Here's how the part is built. I have some questions about the finished solid (model axes, mm). A direction names the side the tool comes from. Round coordinates to 2 decimals unless told otherwise and drop trailing zeros. Loops run counter-clockwise (first coordinate to the right, second up) from the corner with the lowest first, then second, coordinate; pieces in that order, holes last. Notation, with made-up numbers: M 25,9.25 L 71,9.25 A30 cw 71,41.25 Z; hole C -4,57 d9. An arc over 180 degrees is marked long. Answer as a JSON object with one key per item and string values.
from build123d import *

# Parameters (mm, degrees)
EXTRUSION1_DEPTH = 87.5
ESQUISSE3_R      = 1.5
EXTRUSION3_DEPTH = 10
ESQUISSE4_W      = 18.5
ESQUISSE4_H      = 20
EXTRUSION4_DEPTH = 1.5


with BuildPart() as part:
    # Esquisse1 → Extrusion1 (new body)
    with BuildSketch(Plane.XY):
        Polygon((0, 0), (20, 0), (20, 1.5), (1.5, 1.5), (1.5, 20), (0, 20), align=None)
    extrude(amount=EXTRUSION1_DEPTH)

    # Esquisse3 → Extrusion3 (cut)
    with BuildSketch(Plane.ZY):
        with Locations(Location((77.5, 10, 0), (0, 0, 270))):
            Circle(ESQUISSE3_R)
        with Locations(Location((10, 10, 0), (0, 0, 270))):
            Circle(ESQUISSE3_R)
    extrude(amount=-EXTRUSION3_DEPTH, mode=Mode.SUBTRACT)

    # Esquisse4 → Extrusion4 (cut)
    with BuildSketch(Plane.XZ):
        with Locations((10.75, 10)):
            Rectangle(ESQUISSE4_W, ESQUISSE4_H)
        with Locations((10.75, 77.5)):
            Rectangle(ESQUISSE4_W, ESQUISSE4_H)
    extrude(amount=-EXTRUSION4_DEPTH, mode=Mode.SUBTRACT)


solid = part.part
Item 1: For faces 1 (the face through (11, 1, 67.5)), 2 (the face through (20, 1, 43)), 3 (the face through (11, 1, 20)), which set-ups out of +Z, -Z, +X, -X, +Y, -Y let a thin tool reach every point of the face, with its end or its side?
Solution:
{"face 1": "+Z, +X, +Y, -Y", "face 2": "+Z, -Z, +X, +Y, -Y", "face 3": "-Z, +X, +Y, -Y"}
Item 2: I want a section at A-A on y = 10. List the corners of the cut face in (x, z) for me.
Solution:
{"outline": "M 0,0 L 1.5,0 L 1.5,8.5 L 0,8.5 Z; M 0,11.5 L 1.5,11.5 L 1.5,76 L 0,76 Z; M 0,79 L 1.5,79 L 1.5,87.5 L 0,87.5 Z"}
Item 3: I want a section at B-B on z = 77.5. List the corners of the cut face in (x, y) for me, plus the area to 3 significant figures.
Solution:
{"outline": "M 0,0 L 1.5,0 L 1.5,8.5 L 0,8.5 Z; M 0,11.5 L 1.5,11.5 L 1.5,20 L 0,20 Z", "area": "25.5 mm2"}
Item 4: For P1, Ø1.6, axis at x = 7.5, y = 1, coming from the -Z side; P2, Ø4, axis at y = 4, z = 77.5, coming from the +X side; P3, Ø9, axis at x = 8.5, z = 54.5, coming from the +Y side, each with a flat end and sliding along its axis, tell me the tip position at first contact or that it passes through.
Solution:
{"P1": "stops at z = 20", "P2": "stops at x = 1.5", "P3": "stops at y = 1.5"}
Item 5: I want a section at C-C on x = 7.5. List the corners of the cut face in (y, z) for me, plus the area to 4 significant figures.
Solution:
{"outline": "M 0,20 L 1.5,20 L 1.5,67.5 L 0,67.5 Z", "area": "71.25 mm2"}
Item 6: We'd pull the mould along Z, two halves only. Please class faces 4 (the face through (11, 1.5, 43)), 5 (the face through (0.7, 11.2, 9.1)), 6 (the face through (1, 10, 0)): +Z half, -Z half, draft (parallel to the pull), parting line (faces both ways), or undercut.
Solution:
{"face 4": "draft", "face 5": "undercut", "face 6": "-Z half"}
Item 7: I want a section at D-D on z = 14. List the corners of the cut face in (x, y) for me.
Solution:
{"outline": "M 0,0 L 1.5,0 L 1.5,20 L 0,20 Z"}
Item 8: If I drill on L1, parallel to Z at x = 0.3, y = 10; L2, parallel to Y at x = 1, z = 77.5; L3, parallel to X at y = 4, z = 68, over which ranges is the centre line in solid material (lowest first)? Write a range as from..to.
Solution:
{"L1": "z = 0..8.5, 11.5..76, 79..87.5", "L2": "y = 0..8.5, 11.5..20", "L3": "x = 0..1.5"}
